Input: part model. Units: mm. Frame: model coordinates. Face numbers are marked on the shaded views. Give positions to 0.01 mm unless a question says otherwise; leave off trailing zeros. Loops run counter-clockwise (first coordinate to the right, second up) from the corner with the lowest first, then second, coordinate; pieces in that order, holes last. Notation, with made-up numbers: (56.5, 38.5) -> (78.5, 38.5) arc R19 cw to (78.5, 51.5) -> close; hole circle Ø2 at (-2, 3.5). An arc over 180 degrees is marked (long way). Use CSV: the item, a comma, the result in double quotes.
```python
from build123d import *

# Parameters (mm, degrees)
BOSS_EXTRUDE1_DEPTH      = 3
BOSS_EXTRUDE1_DEPTH_BACK = 3
SKETCH3_R                = 3
SKETCH3_R_2              = 2.1
CHAMFER1_SIZE            = 0.09
CHAMFER2_SIZE            = 0.135


with BuildPart() as part:
    # Sketch3 → Boss-Extrude1 (new, two sides: drawn at the far end of the back side and taken through both)
    with BuildSketch(Plane.XY.offset(-BOSS_EXTRUDE1_DEPTH_BACK)):
        Circle(SKETCH3_R)
        Circle(SKETCH3_R_2, mode=Mode.SUBTRACT)
    extrude(amount=BOSS_EXTRUDE1_DEPTH + BOSS_EXTRUDE1_DEPTH_BACK)

    # Chamfer1
    chamfer1_edges = [part.edges().sort_by_distance(p)[0] for p in [
        (-3, 0, -3),
        (-3, 0, 3),
    ]]
    chamfer(chamfer1_edges, length=CHAMFER1_SIZE)

    # Chamfer2
    chamfer2_edges = [part.edges().sort_by_distance(p)[0] for p in [
        (-2.1, 0, -3),
        (-2.1, 0, 3),
    ]]
    chamfer(chamfer2_edges, length=CHAMFER2_SIZE)


solid = part.part
```
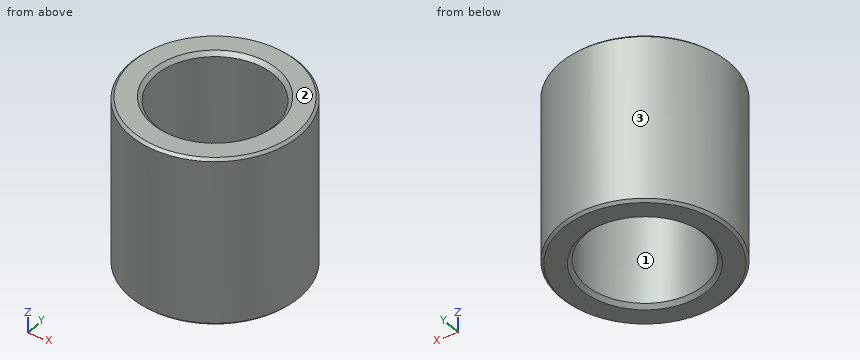
1) Section query A-A (y = 0). Return loops of the section in (x, z) (3 decimals).
From the geometry:
outline,"(-3, -2.91) -> (-2.91, -3) -> (-2.235, -3) -> (-2.1, -2.865) -> (-2.1, 2.865) -> (-2.235, 3) -> (-2.91, 3) -> (-3, 2.91) -> close; (2.1, -2.865) -> (2.235, -3) -> (2.91, -3) -> (3, -2.91) -> (3, 2.91) -> (2.91, 3) -> (2.235, 3) -> (2.1, 2.865) -> close"
2) Mould query, pull axis X, two halves, no side actions, for the marked faces 1, 2 and 3. Classes: pulls with the +X half, pulls with the -X half, needs draft (parallel to the pull), parting line crosses it, or undercut.
From the geometry:
face 1,"undercut"
face 2,"needs draft"
face 3,"parting line crosses it"
3) Section query C-C (z = 0.4). Return loops of the section in (x, y).
From the geometry:
outline,"circle Ø6 at (0, 0); hole circle Ø4.2 at (0, 0)"
4) Ray query, line 1 (Y direction, x = 0, z = -0.7); line 2 (Y direction, x = 1.75, z = 0.4); line 3 (X direction, y = 1.3, z = 0.4). Return the intervals inside material, ascending.
From the geometry:
line 1,"y = -3 to -2.1, 2.1 to 3"
line 2,"y = -2.44 to -1.16, 1.16 to 2.44"
line 3,"x = -2.7 to -1.65, 1.65 to 2.7"
5) Contact query for a flat-ended pin moving along its axis: pin 1 (2 mm diameter, centred on y = 1.5, z = -0.5, fed in from +X). Output: stop coordinate, or through.
From the geometry:
pin 1,"stops at x = 2.96"
